```python
from build123d import *

# Parameters (mm, degrees)
ESBO_O1_R                = 60
RESSALTO_EXTRUS_O1_DEPTH = 9
ESBO_O3_R                = 12
RESSALTO_EXTRUS_O2_DEPTH = 7
ESBO_O4_R                = 1.25
CORTE_EXTRUS_O1_DEPTH    = 10


with BuildPart() as part:
    # Esboço1 → Ressalto-extrusão1 (new body)
    with BuildSketch(Plane.XY):
        Circle(ESBO_O1_R)
        with BuildLine():
            Line((-1.80641219, 2.55), (1.80641219, 2.55))
            ThreePointArc((1.80641219, 2.55), (0, -3.125), (-1.80641219, 2.55))
        make_face(mode=Mode.SUBTRACT)
    extrude(amount=RESSALTO_EXTRUS_O1_DEPTH)

    # Esboço3 → Ressalto-extrusão2 (add)
    with BuildSketch(Plane.XY.offset(9)):
        Circle(ESBO_O3_R)
        with BuildLine():
            Line((-1.80641219, 2.55), (1.80641219, 2.55))
            ThreePointArc((1.80641219, 2.55), (0, -3.125), (-1.80641219, 2.55))
        make_face(mode=Mode.SUBTRACT)
    extrude(amount=RESSALTO_EXTRUS_O2_DEPTH)

    # Esboço4 → Corte-extrusão1 (cut)
    with BuildSketch(Plane.XZ.offset(-2.55)):
        with Locations((0, 13.363805145)):
            Circle(ESBO_O4_R)
    extrude(amount=-CORTE_EXTRUS_O1_DEPTH, mode=Mode.SUBTRACT)


solid = part.part
```
Design review of the part built by this model. Coordinates are the model's own, in mm. A direction names the side the tool comes from. Coordinates: 2 decimals unless noted, no trailing zeros. Loops run counter-clockwise (first coordinate to the right, second up) from the corner with the lowest first, then second, coordinate; pieces in that order, holes last. Notation, with made-up numbers: (-18.75, -17) - (7.25, -17) arc R12 cw to (7.25, 1) - close; hole circle Ø2 at (70, 21.25). An arc over 180 degrees is marked (long way). Use CSV: the item, a comma, the result in double quotes. Start each with the question number.
1) For pin 1 Ø1.8 at (x, z) = (-0.5, 11) entering from -Y; pin 2 Ø6 at (x, y) = (18.5, -31.5) entering from +Z; pin 3 Ø5 at (x, y) = (-28, 10) entering from -Z; pin 4 Ø8 at (y, z) = (-16, 6) entering from +X, all flat-tipped, find the tip position at first contact; note any pin that passes through.
2) Wall thickness on L1, parallel to Y at x = 0, z = 9.5 (3 decimals); L2, parallel to Y at x = 0, z = 7.75 (3 decimals); L3, parallel to Z at x = 0, y = 8.5: over which ranges is each line inside the solid? List them lowest first. Write a range as from..to.
3) Consider section C-C on z = 4.75. Write out the cut boundary in (x, y) (3 decimals).
4) The part is to be moulded in two halves that separate along Y. For faces 3 (the cylindrical face through (-11.99, 0.53, 12.45)), 4 (the cylindrical face through (0.11, -3.123, 7.888)), 5 (the flat face through (12.5, 0.8, 9)), say which applies: +Y half, -Y half, draft (parallel to the pull), parting line (faces both ways), or undercut.
5) Consider section D-D on y = 18.5. Write out the cut boundary in (x, z), then the cut area to 3 significant figures.
6) Tool access review of faces 1 (the flat face through (12, 1, 0)), 2 (the flat face through (0, 2.55, 8)): name each direction out of +Z, -Z, +X, -X, +Y, -Y from which nothing blocks a thin tool from reaching the whole face with its end or side.
7) Consider section A-A on y = 0. Write out the cut boundary in (x, z) (3 decimals), then the cut area to 3 significant figures.
8) Consider section B-B on x = 36. Write out the cut boundary in (y, z), then the cut area to 3 significant figures.
Geometry says:
1,pin 1,"y = -12"
1,pin 2,"z = 9"
1,pin 3,"z = 0"
1,pin 4,"x = 58.79"
2,L1,"-12..-3.125, 2.55..12"
2,L2,"-60..-3.125, 2.55..60"
2,L3,"0..12.11, 14.61..16"
3,outline,"circle Ø120 at (0, 0); hole (-1.806, 2.55) arc R3.125 ccw (long way) to (1.806, 2.55) - close"
4,face 3,"parting line"
4,face 4,"undercut"
4,face 5,"draft"
5,outline,"(-57.08, 0) - (57.08, 0) - (57.08, 9) - (-57.08, 9) - close"
5,area,"1,030 mm^2"
6,face 1,"-Z, +X, -X, +Y, -Y"
6,face 2,"+Z, -Z"
7,outline,"(-60, 0) - (-3.125, 0) - (-3.125, 16) - (-12, 16) - (-12, 9) - (-60, 9) - close; (3.125, 0) - (60, 0) - (60, 9) - (12, 9) - (12, 16) - (3.125, 16) - close"
7,area,"1,150 mm^2"
8,outline,"(-48, 0) - (48, 0) - (48, 9) - (-48, 9) - close"
8,area,"864 mm^2"
